Answer from the drawing. Dimensions are ordinates in mm from the lowest x, y and z of the part. Give positions to 0.01 mm unless a question says otherwise; leave off trailing zeros. Write each loop counter-clockwise with the first axis right and the second up, starting at its lowest first coordinate (ties: lowest second). Pieces come first, ordered by that corner, then holes. Notation, with made-up numbers: M 9.5,68 L 68.5,68 A25 cw 68.5,104 Z; hole C -20.75,11.5 d3. An arc over 180 degrees is marked long. Put each result on its own line as item: value.
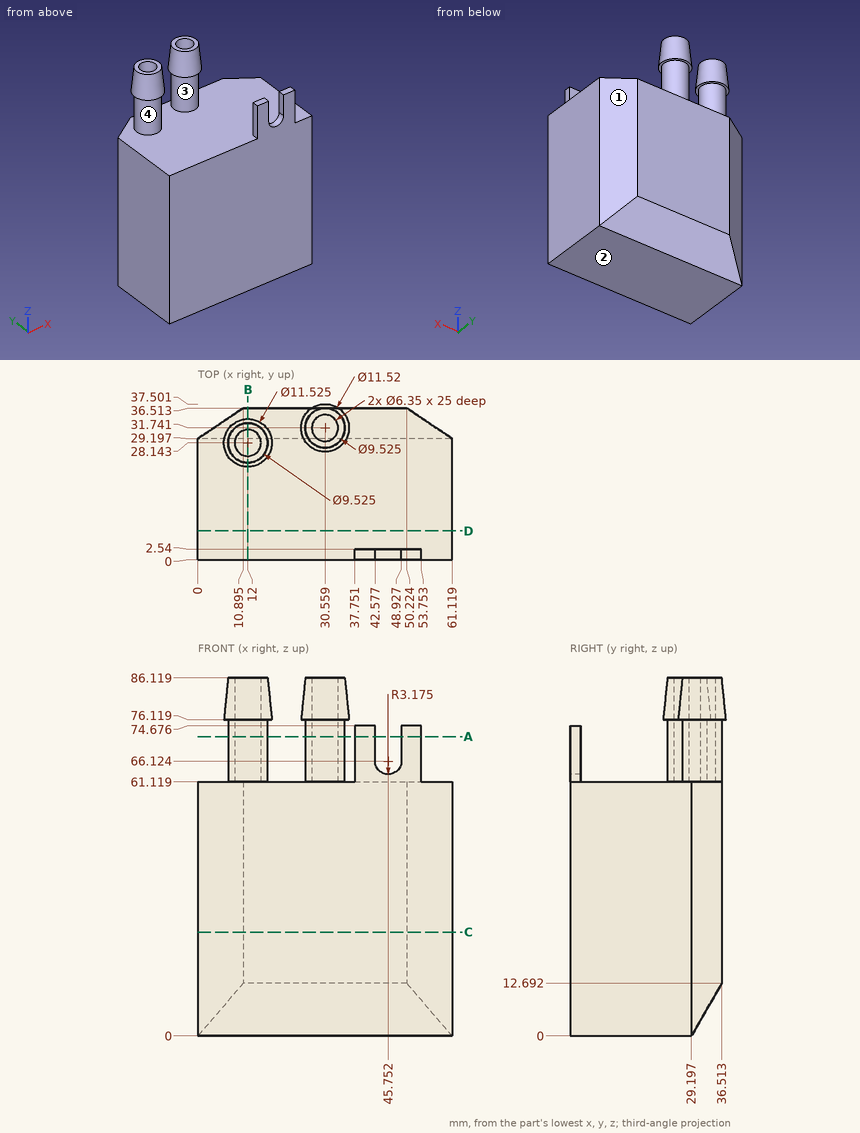
(1) Section B-B on x = 12 is taken. Determine the outline of the cut face in (y, z) (1 decimal).
Result:
outline: M 0,0 L 29.2,0 L 36.5,12.7 L 36.5,61.1 L 32.9,61.1 L 32.9,76.1 L 33.9,76.1 L 32.9,86.1 L 31.3,86.1 L 31.3,61.1 L 25,61.1 L 25,86.1 L 23.4,86.1 L 22.4,76.1 L 23.4,76.1 L 23.4,61.1 L 0,61.1 Z
(2) Section A-A on z = 72 is taken. Give the number of separate pieces and of enclosed holes in the cut face, and give its area (3 significant figures).
Result:
separate pieces: 4
enclosed holes: 2
area: 104 mm²
(3) For a pull along X with two mould halves and no side action, classify the marked faces 1, 2, 3 and 4 as +X half, -X half, draft (parallel to the pull), parting line (faces both ways), or undercut.
Result:
face 1: +X half
face 2: draft
face 3: undercut
face 4: undercut
(4) Given pin 1 Ø6 at (y, z) = (30.5, 37) entering from -X; pin 2 Ø3 at (x, y) = (40, 0.5) entering from +Z; pin 3 Ø0.8 at (y, z) = (1, 68) entering from +X; pin 4 Ø0.8 at (y, z) = (1, 69.5) entering from -X, each flat-ended and moving along its own axis, determine where each tip first touches the part or whether it passes through.
Result:
pin 1: stops at x = 0
pin 2: stops at z = 74.68
pin 3: stops at x = 53.75
pin 4: stops at x = 37.75
(5) Straight lines are drawn through the part: line 1 along Y through (x, z) = (12, 73) (1 decimal); line 2 along Z through (x, y) = (56, 25.5); line 3 along Y through (x, z) = (31, 44). For each, find the intervals that lie inside material, in ascending order. Write a range as from..to.
Result:
line 1: y = 23.4..25, 31.3..32.9
line 2: z = 0..61.12
line 3: y = 0..36.51
(6) Section D-D on y = 7 is taken. Determine the outline of the cut face in (x, z).
Result:
outline: M 0,0 L 61.12,0 L 61.12,61.12 L 0,61.12 Z
(7) Section C-C on z = 25 is taken. Determine the outline of the cut face in (x, y) (1 decimal), and give its area (3 significant figures).
Result:
outline: M 0,0 L 61.1,0 L 61.1,29.2 L 50.2,36.5 L 10.9,36.5 L 0,29.2 Z
area: 2,150 mm²
